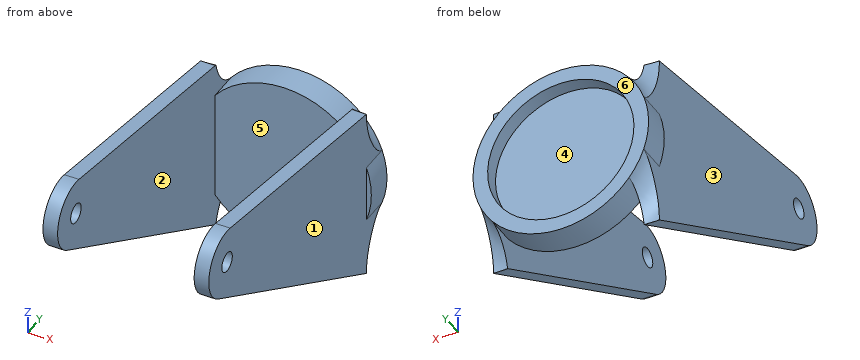
```python
from build123d import *

# Parameters (mm, degrees)
ESQUISSE1_R        = 18
ESQUISSE1_R_2      = 15
BOSS_EXTRU_1_DEPTH = 3
BOSS_EXTRU_3_START = 3
ESQUISSE3_R        = 18
BOSS_EXTRU_3_DEPTH = 3
BOSS_EXTRU_2_START = 14
ESQUISSE2_R        = 2
BOSS_EXTRU_2_DEPTH = 3
FILLET1_R          = 6.6


with BuildPart() as part:
    # Esquisse1 → Boss.-Extru.1 (new body)
    with BuildSketch(Plane(origin=(0, 0, 0), x_dir=(1, 0, 0), z_dir=(0, 1, 0))):
        with Locations(Location((0, 0, 0), (0, 0, 270))):
            Circle(ESQUISSE1_R)
        with Locations(Location((0, 0, 0), (0, 0, 270))):
            Circle(ESQUISSE1_R_2, mode=Mode.SUBTRACT)
    extrude(amount=BOSS_EXTRU_1_DEPTH)

    # Esquisse3 → Boss.-Extru.3 (add)
    with BuildSketch(Plane.XZ.offset(BOSS_EXTRU_3_START)):
        with Locations(Location((0, 0, 0), (0, 0, 270))):
            Circle(ESQUISSE3_R)
    extrude(amount=-BOSS_EXTRU_3_DEPTH)

    # Esquisse2 → Boss.-Extru.2 (add)
    with BuildSketch(Plane(origin=(0, 0, 0), x_dir=(0, 0, -1), z_dir=(1, 0, 0)).offset(BOSS_EXTRU_2_START)):
        with BuildLine():
            Line((-18, -3), (-26.900313921, -55.172856085))
            ThreePointArc((-26.900313921, -55.172856085), (-22.337080841, -62.94833715), (-13.89709797, -59.778496291))
            Line((-13.89709797, -59.778496291), (18, -3))
            Line((18, -3), (-18, -3))
        make_face()
        with Locations((-20, -56.35)):
            Circle(ESQUISSE2_R, mode=Mode.SUBTRACT)
    boss_extru_2 = extrude(amount=BOSS_EXTRU_2_DEPTH)

    # Symétrie1: Boss.-Extru.2 across plane
    add(boss_extru_2.mirror(Plane(origin=(0, 0, 0), x_dir=(0, 0, 1), z_dir=(1, 0, 0))))

    # Fillet1
    # the kernel refuses this fillet: 6.6 mm, written as the material it adds along each edge
    with BuildSketch(Plane(origin=(0, -3, 0), x_dir=(-0.8375611584299304, 0, 0.5463435786110358), z_dir=(0.5463435786110358, 0, 0.8375611584299304))) as fillet1_piece_1_section:
        with BuildLine():
            CenterArc((24.57267069, -6.6), FILLET1_R, 90, 84.78409143)
            Line((24.57267069, 0), (18, 0))
            Line((18, 0), (18, -6))
        make_face()
    fillet1_piece_1 = revolve(axis=Axis((0, -3, 0), (0, -1, 0)), revolution_arc=124.363631706, mode=Mode.PRIVATE)
    fillet1_piece_1 = split(fillet1_piece_1, bisect_by=Plane(origin=(-14, -3, 0), z_dir=(-1, 0, 0)), keep=Keep.TOP, mode=Mode.PRIVATE)
    fillet1_piece_1 = split(fillet1_piece_1, bisect_by=Plane(origin=(-17, -3, 0), z_dir=(1, 0, 0)), keep=Keep.TOP, mode=Mode.PRIVATE)
    fillet1_piece_1 = split(fillet1_piece_1, bisect_by=Plane(origin=(0, -10.686285419, -13.681988516), z_dir=(0, 0.4897851844267101, 0.871843147083289)), keep=Keep.TOP, mode=Mode.PRIVATE)
    add(fillet1_piece_1)
    with BuildSketch(Plane(origin=(0, -3, 0), x_dir=(0.021764364768608612, 0, 0.999763128158975), z_dir=(0.999763128158975, 0, -0.021764364768608612))) as fillet1_piece_2_section:
        with BuildLine():
            CenterArc((24.57267069, -6.6), FILLET1_R, 90, 84.78409143)
            Line((24.57267069, 0), (18, 0))
            Line((18, 0), (18, -6))
        make_face()
    fillet1_piece_2 = revolve(axis=Axis((0, -3, 0), (0, -1, 0)), revolution_arc=124.363631706, mode=Mode.PRIVATE)
    fillet1_piece_2 = split(fillet1_piece_2, bisect_by=Plane(origin=(-14, -3, 0), z_dir=(-1, 0, 0)), keep=Keep.TOP, mode=Mode.PRIVATE)
    fillet1_piece_2 = split(fillet1_piece_2, bisect_by=Plane(origin=(0, -0.016164781, 17.490979177), z_dir=(0, -0.1681634163647939, -0.9857591315308831)), keep=Keep.TOP, mode=Mode.PRIVATE)
    fillet1_piece_2 = split(fillet1_piece_2, bisect_by=Plane(origin=(-17, -3, 0), z_dir=(1, 0, 0)), keep=Keep.TOP, mode=Mode.PRIVATE)
    add(fillet1_piece_2)
    with BuildSketch(Plane(origin=(0, -3, 0), x_dir=(-0.021764364768691844, 0, -0.9997631281589732), z_dir=(-0.9997631281589732, 0, 0.021764364768691844))) as fillet1_piece_3_section:
        with BuildLine():
            CenterArc((24.57267069, -6.6), FILLET1_R, 90, 84.78409143)
            Line((24.57267069, 0), (18, 0))
            Line((18, 0), (18, -6))
        make_face()
    fillet1_piece_3 = revolve(axis=Axis((0, -3, 0), (0, -1, 0)), revolution_arc=124.363631706, mode=Mode.PRIVATE)
    fillet1_piece_3 = split(fillet1_piece_3, bisect_by=Plane(origin=(14, -3, 0), z_dir=(1, 0, 0)), keep=Keep.TOP, mode=Mode.PRIVATE)
    fillet1_piece_3 = split(fillet1_piece_3, bisect_by=Plane(origin=(17, -3, 0), z_dir=(-1, 0, 0)), keep=Keep.TOP, mode=Mode.PRIVATE)
    fillet1_piece_3 = split(fillet1_piece_3, bisect_by=Plane(origin=(0, -10.686285419, -13.681988516), z_dir=(0, 0.4897851844267101, 0.871843147083289)), keep=Keep.TOP, mode=Mode.PRIVATE)
    add(fillet1_piece_3)
    with BuildSketch(Plane(origin=(0, -3, 0), x_dir=(0.8375611584299263, 0, -0.5463435786110422), z_dir=(-0.5463435786110422, 0, -0.8375611584299263))) as fillet1_piece_4_section:
        with BuildLine():
            CenterArc((24.57267069, -6.6), FILLET1_R, 90, 84.78409143)
            Line((24.57267069, 0), (18, 0))
            Line((18, 0), (18, -6))
        make_face()
    fillet1_piece_4 = revolve(axis=Axis((0, -3, 0), (0, -1, 0)), revolution_arc=124.363631706, mode=Mode.PRIVATE)
    fillet1_piece_4 = split(fillet1_piece_4, bisect_by=Plane(origin=(14, -3, 0), z_dir=(1, 0, 0)), keep=Keep.TOP, mode=Mode.PRIVATE)
    fillet1_piece_4 = split(fillet1_piece_4, bisect_by=Plane(origin=(17, -3, 0), z_dir=(-1, 0, 0)), keep=Keep.TOP, mode=Mode.PRIVATE)
    fillet1_piece_4 = split(fillet1_piece_4, bisect_by=Plane(origin=(0, -0.016164781, 17.490979177), z_dir=(0, -0.1681634163647939, -0.9857591315308831)), keep=Keep.TOP, mode=Mode.PRIVATE)
    add(fillet1_piece_4)


solid = part.part
```
The model under review builds one solid part; all positions refer to its coordinate system, in mm. Face numbers are marked on the shaded views. A direction names the side the tool comes from. Give positions to 0.01 mm unless a question says otherwise; leave off trailing zeros. Write each loop counter-clockwise with the first axis right and the second up, starting at its lowest first coordinate (ties: lowest second). Pieces come first, ordered by that corner, then holes. Notation, with made-up numbers: M -12.75,-34.5 L 24.25,-34.5 A34 ccw 24.25,-0.5 Z; hole C 16.25,4.5 d5. An arc over 180 degrees is marked long. Write item = value, one per line. Start each with the question number.
Q1. We need section A-A (x = 0). State the section outline as (y, z) points.
Q2. Clearance check with flat-ended pins moving along their axes: pin 1 (15 mm diameter, centred on x = 0, z = -4.5, fed in from +Y); pin 2 (3 mm diameter, centred on y = -17.5, z = 6.5, fed in from -X); pin 3 (5 mm diameter, centred on x = 10.5, z = -9, fed in from -Y). State where each tip first meets the part, or that it passes through.
Q3. We need section D-D (y = -56.35). State the section outline as (x, z) points, plus the area to 3 significant figures.
Q4. Machinability: for the marked faces 5 and 6, which of the approach directions +Z, -Z, +X, -X, +Y, -Y give a long, thin tool a straight path to every point of the face, cutting with its end or side? Answer none if there is none.
Q5. We need section B-B (y = -9.5). State the section outline as (x, z) points.
Q6. Mouldability with a two-part tool opening along X and no side actions: class the marked faces 1, 2, 3 and 4 as released by +X, released by -X, zero draft, split by the parting line, or undercut.
Q7. For line 1 (X direction, y = 1, z = 0); line 2 (X direction, y = -46, z = 7.5); line 3 (Y direction, x = -10.5, z = -1.5), list the stretches that pass through material, from the lowest coordinate up.
Q8. We need section C-C (z = 21). State the section outline as (x, y) points.
Result set:
q1.outline = M -3,-18 L 3,-18 L 3,-15 L 0,-15 L 0,15 L 3,15 L 3,18 L -3,18 Z
q2.pin_1 = 0
q2.pin_2 = -17
q2.pin_3 = -3
q3.outline = M -17,11.97 L -14,11.97 L -14,18 L -17,18 Z; M -17,22 L -14,22 L -14,27 L -17,27 Z; M 14,11.97 L 17,11.97 L 17,18 L 14,18 Z; M 14,22 L 17,22 L 17,27 L 14,27 Z
q3.area = 66.2 mm2
q4.face_5 = +Z, -Z, -Y
q4.face_6 = +Z, -Z, +X, -X, +Y
q5.outline = M -17,-14.35 L -14,-14.35 L -14,19.11 L -17,19.11 Z; M 14,-14.35 L 17,-14.35 L 17,19.11 L 14,19.11 Z
q6.face_1 = released by +X
q6.face_2 = undercut
q6.face_3 = released by -X
q6.face_4 = undercut
q7.line_1 = -18 to -15, 15 to 18
q7.line_2 = -17 to -14, 14 to 17
q7.line_3 = -3 to 0
q8.outline = M -17,-63.28 L -14,-63.28 L -14,-58.08 L -17,-58.08 Z; M -17,-54.62 L -14,-54.62 L -14,-20.59 L -17,-20.59 Z; M 14,-63.28 L 17,-63.28 L 17,-58.08 L 14,-58.08 Z; M 14,-54.62 L 17,-54.62 L 17,-20.59 L 14,-20.59 Z
